Design review of the part built by this model. Coordinates are the model's own, in mm. Coordinates: 2 decimals unless noted, no trailing zeros. Write each loop counter-clockwise with the first axis right and the second up, starting at its lowest first coordinate (ties: lowest second). Pieces come first, ordered by that corner, then holes. Notation, with made-up numbers: (-22, -28) - (36, -28) arc R24 cw to (36, -16) - close; hole circle Ø10 at (64, 63.5). An arc over 180 degrees is marked (long way). Answer as a JSON object with one key per item and string values.
Solid Edge part; units mm, degrees
sketch "Sketch1" plane through (0, 0, 0) normal (0, 0, 1) x (1, 0, 0)
  line L0 (-3.5, 2.0207) -> (-3.5, -2.0207)
  line L1 (-3.5, -2.0207) -> (0, -4.0415)
  line L2 (0, -4.0415) -> (3.5, -2.0207)
  line L3 (3.5, -2.0207) -> (3.5, 2.0207)
  line L4 (3.5, 2.0207) -> (0, 4.0415)
  line L5 (0, 4.0415) -> (-3.5, 2.0207)
extrude "Protrusion1" add sketch "Sketch1" along normal blind 3.2
hole "Hole1" at (0, 0, 3.2) direction (0, 0, -1) diameter 3.242 end up to next
sketch "Sketch2" plane through (0, 0, 0) normal (1, 0, 0) x (0, 1, 0)
  line L0 (3.5, 3.2) -> (4.0415, 3.0029)
revolve "RevolvedCutout1" cut sketch "Sketch2" angle 360 about axis through (0, 0, -60.325) along (0, 0, 1) material side at (0, 3.7879, 3.1484)
sketch "Sketch3" plane through (0, 0, 0) normal (1, 0, 0) x (0, 1, 0)
  line L0 (4.0415, 0.1971) -> (3.5, 0)
revolve "RevolvedCutout2" cut sketch "Sketch3" angle 360 about axis through (0, 0, -60.325) along (0, 0, 1) material side at (0, 3.7879, 0.0516)
properties part number "062"
(1) The part is to be moulded in two halves that separate along Z. For faces 1 (the face through (1.8, 3, 1.6)), 2 (the face through (1, -2, 0)), 3 (the face through (0.08, -3.652, 3.144)), say which applies: pulls with the +Z half, pulls with the -Z half, needs draft (parallel to the pull), parting line crosses it, or undercut.
Solved:
{"face 1": "needs draft", "face 2": "pulls with the -Z half", "face 3": "pulls with the +Z half"}
(2) Take a section at A-A, the plane z = 2.6. Write out the cut boundary in (x, y), and give its area (3 significant figures).
Solved:
{"outline": "(-3.5, -2.02) - (0, -4.04) - (3.5, -2.02) - (3.5, 2.02) - (0, 4.04) - (-3.5, 2.02) - close; hole circle Ø3.24 at (0, 0)", "area": "34.2 mm^2"}
(3) To check wall thickness, follow line 1 (X direction, y = 0, z = 1.75); line 2 (Y direction, x = -0.25, z = 2.3); line 3 (X direction, y = 0.75, z = 2.75). State the ranges of each line that lie inside material, in increasing order. Write a range as from..to.
Solved:
{"line 1": "x = -3.5..-1.62, 1.62..3.5", "line 2": "y = -3.9..-1.6, 1.6..3.9", "line 3": "x = -3.5..-1.44, 1.44..3.5"}
